Check sheet for the drawn part. Datum: minimum x, y, z corner. Units: mm. A direction names the side the tool comes from. Give positions to 0.01 mm unless a question says otherwise; leave off trailing zeros. Order: outer loops, then holes, each group sorted by start corner. A loop starts at its lowest first (then second) coordinate and runs counter-clockwise, first axis right, second up.
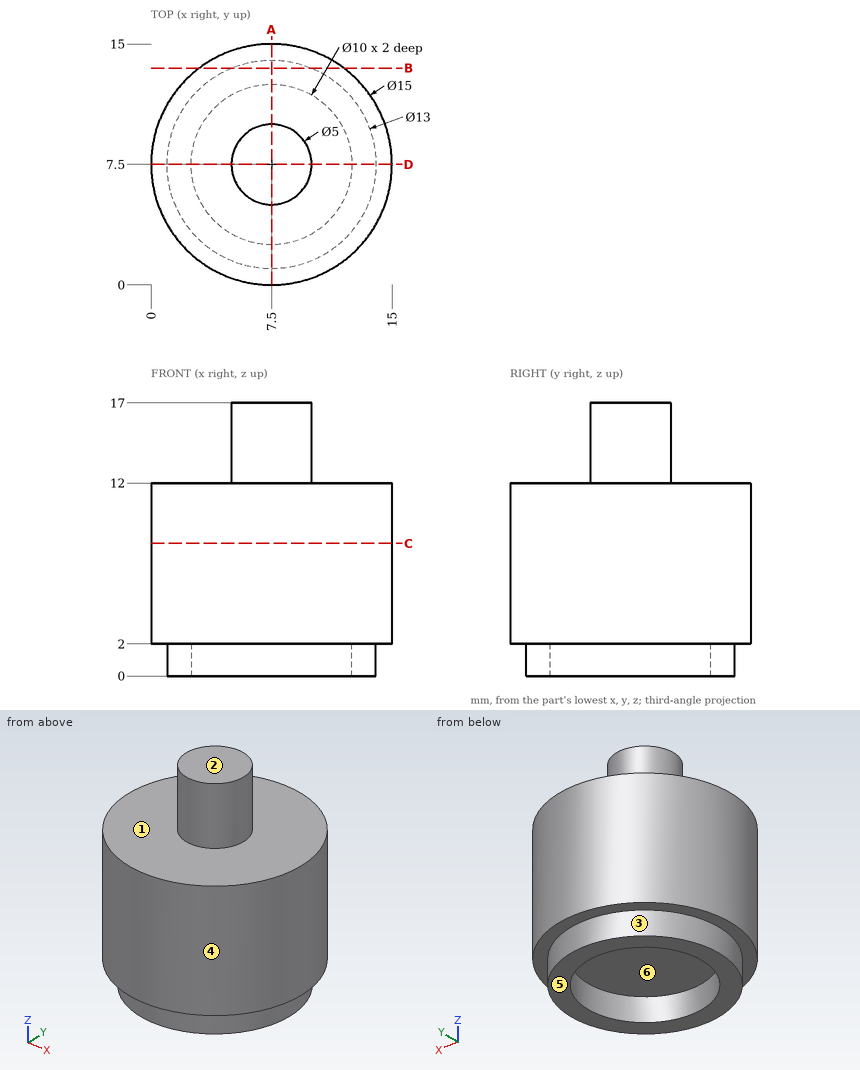
Item 1: Scan lines: L1, parallel to Y at x = 7.5, z = 0.95; L2, parallel to Z at x = 10, y = 10.5; L3, parallel to X at y = 7.25, z = 6. Record each from-to range of solid material in increasing order.
Reported:
L1: y = 1 to 2.5, 12.5 to 14
L2: z = 2 to 12
L3: x = 0 to 15
Item 2: Set-up check for the marked faces 1, 2 and 3: record each of +Z, -Z, +X, -X, +Y, -Y from which the full face is reachable in a straight line by a thin tool's end or side.
Reported:
face 1: +Z
face 2: +Z, +X, -X, +Y, -Y
face 3: -Z
Item 3: Sectioned sample at B-B (y = 13.5). Enter the section's corners in (x, z), and give its area (3 significant figures).
Reported:
outline: (3, 2) - (5, 2) - (5, 0) - (10, 0) - (10, 2) - (12, 2) - (12, 12) - (3, 12) - close
area: 100 mm2
Item 4: Draft check along X on the marked faces 4, 5 and 6. Enter one of: released by +X, released by -X, zero draft, split by the parting line, or undercut.
Reported:
face 4: split by the parting line
face 5: zero draft
face 6: undercut
Item 5: Sectioned sample at C-C (z = 8.25). Enter the section's corners in (x, y).
Reported:
outline: circle Ø15 at (7.5, 7.5)
Item 6: Gauge pin test, flat ends, axial feed: pin 1 (2 mm diameter, centred on y = 13, z = 7.5, fed in from -X); pin 2 (5 mm diameter, centred on x = 5.5, y = 7, fed in from -Z); pin 3 (1.5 mm diameter, centred on x = 11.5, z = 10.5, fed in from -Y). Record the tip position at first contact, or that the pin passes through.
Reported:
pin 1: stops at x = 1.5
pin 2: stops at z = 2
pin 3: stops at y = 0.74
Item 7: Sectioned sample at A-A (x = 7.5). Enter the section's corners in (y, z).
Reported:
outline: (0, 2) - (1, 2) - (1, 0) - (2.5, 0) - (2.5, 2) - (12.5, 2) - (12.5, 0) - (14, 0) - (14, 2) - (15, 2) - (15, 12) - (10, 12) - (10, 17) - (5, 17) - (5, 12) - (0, 12) - close
